CAD build for the part. Positions are in the model's coordinates, mm. Coordinates: 2 decimals unless noted, no trailing zeros. Order: outer loops, then holes, each group sorted by start corner. A loop starts at its lowest first (then second) coordinate and runs counter-clockwise, first axis right, second up. Notation, with made-up numbers: (75, 2.25) - (90, 2.25) arc R26 ccw to (90, 20.25) - close; hole circle Ø10 at (12, 80). An arc over 180 degrees is marked (long way). Write each question's results on one line, items separated by ' | '. Start each with the question number.
Q1. Band-saw the part on A-A, the plane x = 33. Write the cut outline in (y, z).
Q2. Band-saw the part on B-B, the plane y = 35. Write the cut outline in (x, z).
Q3. Pull direction X, two halves, no side cores. Call faces 1 (the cylindrical face through (33.46, 85.72, 25.49)), 2 (the cylindrical face through (37.878, 13.035, 23.409)), 3 (the flat face through (45, 47, 17)), 4 (the flat face through (66, 46, 15)): released by +X, released by -X, zero draft, split by the parting line, or undercut.
Q4. Band-saw the part on C-C, the plane z = 26. Write the cut outline in (x, y), then the cut area to 3 significant figures.
Q5. Pin check, flat tips, straight feed: P1, Ø22.5, axis at x = 27, y = 26.5, coming from the +Z side; P2, Ø1.5, axis at x = 7, z = 14.5, coming from the -Y side; P3, Ø11.5, axis at y = 75, z = 15, coming from the +X side. Stop position of each tip, or through.
Q6. Band-saw the part on D-D, the plane x = 20. Write the cut outline in (y, z), then the cut area to 3 significant figures.
Q7. Wall check: probe 1 along Y at (x, z) = (33, 9); probe 2 along Y at (x, z) = (25.5, 17.5); probe 3 along Y at (x, z) = (26, 26). Give the ranges that are in metal, low to high.
```python
from build123d import *

# Parameters (mm, degrees)
BOSS_EXTRUDE1_DEPTH = 30
SKETCH2_R           = 16.5
CUT_EXTRUDE1_DEPTH  = 17
CUT_EXTRUDE2_REACH  = 15
SKETCH3_R           = 22.5
FILLET2_R           = 15
CUT_EXTRUDE3_REACH  = 68
SKETCH4_R           = 6.5


with BuildPart() as part:
    # Sketch1 → Boss-Extrude1 (new body)
    with BuildSketch(Plane.XY):
        with BuildLine():
            Line((0, 0), (0, 90))
            Line((0, 90), (66, 90))
            Line((66, 90), (66, 0))
            ThreePointArc((66, 0), (33, -4.836485169), (0, 0))
        make_face()
    extrude(amount=BOSS_EXTRUDE1_DEPTH)

    # Sketch2 → Cut-Extrude1 (cut)
    with BuildSketch(Plane(origin=(0, 0, 0), x_dir=(-1, 0, 0), z_dir=(0, 0, -1))):
        with Locations((-33, 35)):
            Circle(SKETCH2_R)
    extrude(amount=-CUT_EXTRUDE1_DEPTH, mode=Mode.SUBTRACT)

    # Sketch3 → Cut-Extrude2 (cut, up to next)
    with BuildSketch(Plane(origin=(0, 0, 17), x_dir=(-1, 0, 0), z_dir=(0, 0, -1)), mode=Mode.PRIVATE) as cut_extrude2_sk1:
        with Locations((-33, 35)):
            Circle(SKETCH3_R)
    cut_extrude2_tool1 = extrude(cut_extrude2_sk1.sketch, amount=-CUT_EXTRUDE2_REACH, mode=Mode.PRIVATE) & part.part
    add(cut_extrude2_tool1.solids().sort_by_distance((33, 35, 17))[0], mode=Mode.SUBTRACT)

    # Fillet2
    fillet2_edges = [part.edges().sort_by_distance(p)[0] for p in [
        (33, 90, 30),
    ]]
    fillet(fillet2_edges, radius=FILLET2_R)

    # Sketch4 → Cut-Extrude3 (cut, up to next)
    with BuildSketch(Plane.ZY, mode=Mode.PRIVATE) as cut_extrude3_sk1:
        with Locations((15, 75)):
            Circle(SKETCH4_R)
    cut_extrude3_tool1 = extrude(cut_extrude3_sk1.sketch, amount=-CUT_EXTRUDE3_REACH, mode=Mode.PRIVATE) & part.part
    add(cut_extrude3_tool1.solids().sort_by_distance((0, 75, 15))[0], mode=Mode.SUBTRACT)


solid = part.part
```
Results below:
1) outline: (-4.84, 0) - (18.5, 0) - (18.5, 17) - (12.5, 17) - (12.5, 30) - (-4.84, 30) - close; (51.5, 0) - (90, 0) - (90, 15) arc R15 ccw to (75, 30) - (57.5, 30) - (57.5, 17) - (51.5, 17) - close; hole circle Ø13 at (75, 15)
2) outline: (0, 0) - (16.5, 0) - (16.5, 17) - (10.5, 17) - (10.5, 30) - (0, 30) - close; (49.5, 0) - (66, 0) - (66, 30) - (55.5, 30) - (55.5, 17) - (49.5, 17) - close
3) face 1: zero draft | face 2: undercut | face 3: undercut | face 4: released by +X
4) outline: (0, 0) arc R115 ccw to (66, 0) - (66, 85.2) - (0, 85.2) - close; hole circle Ø45 at (33, 35) | area: 4,250 mm²
5) P1: stops at z = 17 | P2: stops at y = -2.03 | P3: passes through
6) outline: (-4.1, 0) - (24.84, 0) - (24.84, 17) - (16.64, 17) - (16.64, 30) - (-4.1, 30) - close; (45.16, 0) - (90, 0) - (90, 15) arc R15 ccw to (75, 30) - (53.36, 30) - (53.36, 17) - (45.16, 17) - close; hole circle Ø13 at (75, 15) | area: 1,820 mm²
7) probe 1: y = -4.84 to 18.5, 51.5 to 72.5, 77.5 to 90 | probe 2: y = -4.59 to 13.79, 56.21 to 69, 81 to 89.79 | probe 3: y = -4.62 to 13.62, 56.38 to 85.2
